For this review, take the finished solid that the model builds, in its own axes (mm). A direction names the side the tool comes from. Give positions to 0.01 mm unless a question says otherwise; leave off trailing zeros. Order: outer loops, then holes, each group sorted by start corner. A loop starts at its lowest first (then second) coordinate and runs counter-clockwise, first axis right, second up. Notation, with made-up numbers: (80.25, -22) - (98.25, -22) arc R37 cw to (98.25, 14) - close; hole circle Ø8 at (-12.5, 14). An arc over 180 degrees is marked (long way). Use a Markdown table: item, result. Add a question column.
1) Mouldability with a two-part tool opening along Y and no side actions: class faces 1 (the face through (41.7, 106.3, 102)), 2 (the face through (2.281, 105.594, 103.658)), 3 (the face through (53, 106, 104)) as released by +Y, released by -Y, zero draft, split by the parting line, or undercut.
2) Wall thickness on L1, parallel to Y at x = 8, z = 104.75; L2, parallel to Y at x = 78, z = 102.8: over which ranges is each line inside the solid? List them lowest first.
3) Machinability: for faces 4 (the face through (53, 2, 104)), 5 (the face through (0, 53, 104)), 6 (the face through (8, 8, 103)), which of the approach directions +Z, -Z, +X, -X, +Y, -Y give a long, thin tool a straight path to every point of the face, cutting with its end or side? Answer none if there is none.
4) We need section B-B on z = 104.35. Write out the cut boundary in (x, y).
5) Clearance check with a flat-ended pin moving along its axis: P1, Ø6, axis at x = 8, y = 100, coming from the +Z side. State where the tip first meets the part, or that it passes through.
6) We need section A-A on y = 78.5. Write out the cut boundary in (x, z).
```python
from build123d import *

# Parameters (mm, degrees)
SKETCH128_W     = 108
SKETCH128_H     = 108
PAD051_DEPTH    = 3.27
FILLET010_R     = 8
SKETCH129_R     = 3.25
POCKET051_DEPTH = 2.27
POCKET050_DEPTH = 3.271


with BuildPart() as part:
    # Sketch128 → Pad051 (new body)
    with BuildSketch(Plane.XY):
        with Locations((54, 54)):
            Rectangle(SKETCH128_W, SKETCH128_H)
    extrude(amount=PAD051_DEPTH)

    # Fillet010
    fillet010_edges = [part.edges().sort_by_distance(p)[0] for p in [
        (108, 0, 1.635),
        (108, 108, 1.635),
        (0, 108, 1.635),
        (0, 0, 1.635),
    ]]
    fillet(fillet010_edges, radius=FILLET010_R)

    # Sketch129 (on Face5 of Fillet010) → Pocket051 (cut)
    with BuildSketch(Plane.XY.offset(3.27)):
        with Locations((8, 8)):
            Circle(SKETCH129_R)
        with Locations((100, 8)):
            Circle(SKETCH129_R)
        with Locations((100, 100)):
            Circle(SKETCH129_R)
        with Locations((8, 100)):
            Circle(SKETCH129_R)
    extrude(amount=-POCKET051_DEPTH, mode=Mode.SUBTRACT)

    # Sketch130 (on Face5 of Pocket051) → Pocket050 (cut, through all)
    with BuildSketch(Plane.XY.offset(3.27)):
        with BuildLine():
            Line((2, 94.708497), (2, 13.291503))
            ThreePointArc((13.291503, 2), (13.655204, 13.655204), (2, 13.291503))
            Line((13.291503, 2), (94.708497, 2))
            ThreePointArc((106, 13.291503), (94.343146, 13.656854), (94.708497, 2))
            Line((106, 94.708497), (106, 13.291503))
            ThreePointArc((94.708497, 106), (94.342737, 94.342737), (106, 94.708497))
            Line((13.291503, 106), (94.708497, 106))
            ThreePointArc((2, 94.708497), (13.656854, 94.343146), (13.291503, 106))
        make_face()
    extrude(amount=-POCKET050_DEPTH, mode=Mode.SUBTRACT)


with BuildPart() as part_1:
    # Body023 placement: moved
    add(part.part.moved(Location((0, 0, 102))))


solid = part_1.part
```
Checked values:
| question | item | result |
|---|---|---|
| 1 | face 1 | zero draft |
| 1 | face 2 | released by +Y |
| 1 | face 3 | undercut |
| 2 | L1 | 0 to 4.75, 11.25 to 16, 92 to 96.75, 103.25 to 108 |
| 2 | L2 | 0 to 2, 106 to 108 |
| 3 | face 4 | +Z, -Z |
| 3 | face 5 | +Z, -Z, -X, +Y, -Y |
| 3 | face 6 | +Z |
| 4 | outline | (0, 8) arc R8 ccw to (8, 0) - (100, 0) arc R8 ccw to (108, 8) - (108, 100) arc R8 ccw to (100, 108) - (8, 108) arc R8 ccw to (0, 100) - close; hole (2, 13.29) arc R8 cw (long way) to (13.29, 2) - (94.71, 2) arc R8 cw (long way) to (106, 13.29) - (106, 94.71) arc R8 cw (long way) to (94.71, 106) - (13.29, 106) arc R8 cw (long way) to (2, 94.71) - close; hole circle Ø6.5 at (8, 8); hole circle Ø6.5 at (8, 100); hole circle Ø6.5 at (100, 8); hole circle Ø6.5 at (100, 100) |
| 5 | P1 | z = 103 |
| 6 | outline | (0, 102) - (2, 102) - (2, 105.27) - (0, 105.27) - close; (106, 102) - (108, 102) - (108, 105.27) - (106, 105.27) - close |
